from build123d import *

# Parameters (mm, degrees)
F1_DEPTH = 63.5
F0_W     = 38.328622
F0_H     = 4.7498
F0_H_2   = 4.7752
F0_H_3   = 19.05
F2_DEPTH = 25.4
F3_DEPTH = 7.9375
F5_R     = 5.08


with BuildPart() as f1:
    # F0 (on Front) → F1 (new body, symmetric)
    with BuildSketch(Plane.XZ):
        Polygon((22.225, 9.525), (-41.275, 9.525), (-41.275, -9.525), (41.275, -9.525), (41.275, 9.525), align=None)
    extrude(amount=F1_DEPTH, both=True)

    # F0 (on Front) → F2 (join, symmetric)
    with BuildSketch(Plane.XZ):
        Polygon((22.225, 9.525), (-41.275, 9.525), (-41.275, -9.525), (41.275, -9.525), (41.275, 9.525), align=None)
        with Locations((79.489311, 64.3001)):
            Rectangle(F0_W, F0_H)
        with Locations((79.489311, 40.4876)):
            Rectangle(F0_W, F0_H_2)
        with BuildLine():
            Line((22.225, 27.0002), (22.225, 9.525))
            Line((22.225, 9.525), (41.275, 9.525))
            Line((41.275, 9.525), (41.275, 27.0002))
            ThreePointArc((41.275, 27.0002), (45.92468, 38.22552), (57.15, 42.8752))
            Line((57.15, 42.8752), (60.325, 42.8752))
            Line((60.325, 42.8752), (60.325, 61.9252))
            Line((60.325, 61.9252), (57.15, 61.9252))
            ThreePointArc((57.15, 61.9252), (32.454296, 51.695904), (22.225, 27.0002))
        make_face()
        with Locations((79.489311, 52.4002)):
            Rectangle(F0_W, F0_H_3)
    extrude(amount=F2_DEPTH, both=True)

    # F0 (on Front) → F3 (join, symmetric)
    with BuildSketch(Plane.XZ):
        with BuildLine():
            add(Edge.make_bspline(
                [(-41.275, 9.525), (-32.633623, 51.821707), (19.34902, 67.917436), (60.325, 61.9252)],
                knots=[0, 0, 0, 0, 114.316845, 114.316845, 114.316845, 114.316845], degree=3))
            Line((-41.275, 9.525), (22.225, 9.525))
            Line((22.225, 9.525), (22.225, 27.0002))
            ThreePointArc((22.225, 27.0002), (32.454296, 51.695904), (57.15, 61.9252))
            Line((57.15, 61.9252), (60.325, 61.9252))
        make_face()
    extrude(amount=F3_DEPTH, both=True)

    # F0 (on Front) → F4 (revolve)
    with BuildSketch(Plane.XZ):
        Polygon((98.653622, 66.675), (98.653622, 61.9252), (98.653622, 42.8752), (98.653622, 38.1), (111.125, 38.1), (111.125, 66.675), align=None)
    revolve(axis=Axis((98.653622, 0, 52.3875), (0, 0, 1)))

    # F5
    f5_edges = [f1.edges().sort_by_distance(p)[0] for p in [
        (-41.275, -63.5, 0),
        (41.275, -63.5, 0),
        (41.275, 63.5, 0),
        (-41.275, 63.5, 0),
    ]]
    fillet(f5_edges, radius=F5_R)


solid = f1.part
Part model, mm, in its own coordinate system. A direction names the side the tool comes from. Round coordinates to 2 decimals unless told otherwise and drop trailing zeros. Write each loop counter-clockwise with the first axis right and the second up, starting at its lowest first coordinate (ties: lowest second). Pieces come first, ordered by that corner, then holes. Notation, with made-up numbers: (79, 61) - (84, 61) arc R36 cw to (84, 95) - close; hole circle Ø7 at (9.5, 16). An arc over 180 degrees is marked (long way). Use CSV: the item, a comma, the result in double quotes.
Item 1: Tool access for faces 1 (the flat face through (60, 25.4, 45)), 2 (the flat face through (60.325, 0, 40)), 3 (the flat face through (22.225, -17, 18)), 4 (the flat face through (80, 0, 38.1)): list every direction of +Z, -Z, +X, -X, +Y, -Y with a clear straight run to the whole face (end or side of a thin tool).
Results list:
face 1,"+Z, +X, -X, +Y"
face 2,"-Z, +Y, -Y"
face 3,"+Z, -X, -Y"
face 4,"-Z, +X, +Y, -Y"
Item 2: Pull direction X, two halves, no side cores. Call faces 5 (the flat face through (98.654, 19, 52)), 6 (the cylindrical face through (45.8, -0.4, 38.1)), 7 (the flat face through (1, 35, 9.525)), 8 (the flat face through (-41.275, -1, 0)): pulls with the +X half, pulls with the -X half, needs draft (parallel to the pull), parting line crosses it, or undercut.
Results list:
face 5,"pulls with the +X half"
face 6,"undercut"
face 7,"needs draft"
face 8,"pulls with the -X half"
Item 3: Slice it at B-B, the plane y = 51. Write the cut outline in (x, z) (3 decimals).
Results list:
outline,"(-41.275, -9.525) - (41.275, -9.525) - (41.275, 9.525) - (-41.275, 9.525) - close"
Item 4: Wall check: L1, parallel to Y at x = -3, z = 22; L2, parallel to Z at x = 98.5, y = 1.5 (3 decimals); L3, parallel to Z at x = -15, y = -11 (3 decimals). Give the ranges that are in metal, low to high.
Results list:
L1,"y = -7.94 to 7.94"
L2,"z = 38.1 to 66.675"
L3,"z = -9.525 to 9.525"
Item 5: Flat gauge pins, fed straight in: P1, Ø3, axis at x = 63.5, z = 41.5, coming from the +Y side; P2, Ø6, axis at x = 46.5, z = 8, coming from the +Y side; P3, Ø8, axis at y = 40, z = 4, coming from the +X side (3 decimals); P4, Ø5.5, axis at y = -3.5, z = 40, coming from the -X side. Where does each tip first touch, or does it go through?
Results list:
P1,"stops at y = 25.4"
P2,"passes through"
P3,"stops at x = 41.275"
P4,"stops at x = -26.72"
Item 6: Slice it at A-A, the plane y = 20. Write the cut outline in (x, z) (3 decimals), then the cut area to 3 significant figures.
Results list:
outline,"(-41.275, -9.525) - (41.275, -9.525) - (41.275, 27) arc R15.875 cw to (57.15, 42.875) - (60.325, 42.875) - (60.325, 38.1) - (98.654, 38.1) - (98.654, 66.675) - (60.325, 66.675) - (60.325, 61.925) - (57.15, 61.925) arc R34.925 ccw to (22.225, 27) - (22.225, 9.525) - (-41.275, 9.525) - close"
area,"3,820 mm²"
